Input: dimensioned drawing with shaded views. Units: mm. Origin: part minimum x, y, z. A direction names the side the tool comes from. Give positions to 0.01 mm unless a question says otherwise; leave off trailing zeros. Order: outer loops, then holes, each group sorted by start corner. A loop starts at its lowest first (then second) coordinate and runs counter-clockwise, first axis right, second up. Notation, with made-up numbers: M 46,-18.5 L 63,-18.5 A21 ccw 63,4.5 Z; hole C -3.5,72 d7. An arc over 180 degrees is marked long. Answer in a Markdown table with one row per item. Add a question column.
(1) Section query A-A, the plane z = 6. Return loops of the section in (x, y), plus the area to 3 significant figures.
(2) Material intervals for line 1 along Z through (x, y) = (17.25, 64.5); line 2 along Y through (x, z) = (15, 22.5); line 3 along Y through (x, z) = (15.75, 53.5), sorted ascending.
(3) Mould query, pull axis Z, two halves, no side actions, for the marked faces 4, 5, 6 and 7. Classes: pulls with the +Z half, pulls with the -Z half, needs draft (parallel to the pull), parting line crosses it, or undercut.
(4) Section query B-B, the plane x = 17. Return loops of the section in (y, z), plus the area to 3 significant figures.
(5) Set-up query: the marked faces 1, 2 and 3. Return all of +Z, -Z, +X, -X, +Y, -Y with unobstructed straight access to the full face (end or side cutting, diameter ignored); none if empty.
(6) Section query D-D, the plane x = 7.5. Return loops of the section in (y, z) (1 decimal), plus the area to 3 significant figures.
(7) Section query C-C, the plane y = 83.5. Return loops of the section in (x, z), plus the area to 3 significant figures.
(8) Pin query (flat end, axial travel): P1, Ø6, axis at x = 4.5, y = 77, coming from the +Z side; P2, Ø3, axis at y = 109.5, z = 63, coming from the -X side; P3, Ø2, axis at y = 88.5, z = 37.5, coming from the -X side; P4, Ø6, axis at x = 8, z = 62.5, coming from the -Y side. Return the tip coordinate at first contact, or that it passes through.
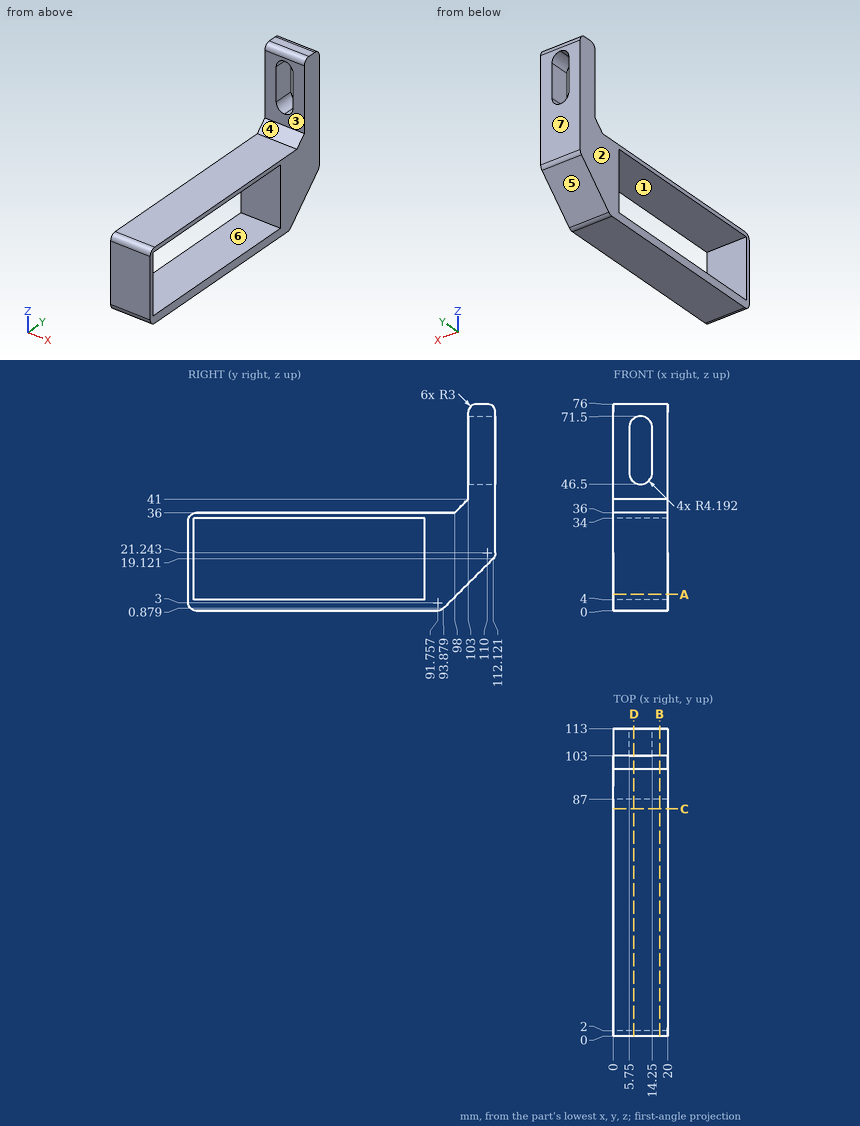
Values follow:
| question | item | result |
|---|---|---|
| 1 | outline | M 0,0 L 20,0 L 20,2 L 0,2 Z; M 0,87 L 20,87 L 20,99 L 0,99 Z |
| 1 | area | 280 mm² |
| 2 | line 1 | z = 0 to 4, 34 to 36 |
| 2 | line 2 | y = 0 to 2, 87 to 113 |
| 2 | line 3 | y = 103 to 113 |
| 3 | face 4 | pulls with the +Z half |
| 3 | face 5 | pulls with the -Z half |
| 3 | face 6 | undercut |
| 3 | face 7 | needs draft |
| 4 | outline | M 0,3 A3 ccw 3,0 L 91.76,0 A3 ccw 93.88,0.88 L 112.12,19.12 A3 ccw 113,21.24 L 113,73 A3 ccw 110,76 L 106,76 A3 ccw 103,73 L 103,41 L 98,36 L 3,36 A3 ccw 0,33 Z; hole M 2,4 L 87,4 L 87,34 L 2,34 Z |
| 4 | area | 1,720 mm² |
| 5 | face 1 | +X, -X |
| 5 | face 2 | +Z, -Z, -X, +Y, -Y |
| 5 | face 3 | +Z, +X, -X, -Y |
| 6 | outline | M 0,3 A3 ccw 3,0 L 91.8,0 A3 ccw 93.9,0.9 L 112.1,19.1 A3 ccw 113,21.2 L 113,47.3 L 103,47.3 L 103,41 L 98,36 L 3,36 A3 ccw 0,33 Z; M 103,70.7 L 113,70.7 L 113,73 A3 ccw 110,76 L 106,76 A3 ccw 103,73 Z; hole M 2,4 L 87,4 L 87,34 L 2,34 Z |
| 6 | area | 1,490 mm² |
| 7 | outline | M 0,0 L 20,0 L 20,4 L 0,4 Z; M 0,34 L 20,34 L 20,36 L 0,36 Z |
| 7 | area | 120 mm² |
| 8 | P1 | stops at z = 36 |
| 8 | P2 | stops at x = 0 |
| 8 | P3 | passes through |
| 8 | P4 | stops at y = 103 |
